```python
from build123d import *

# Parameters (mm, degrees)
SKETCH_1_R      = 1.5
SKETCH_1_R_2    = 1
EXTRUDE_1_DEPTH = 2


with BuildPart() as part:
    # 草图1 → 凸台-拉伸1 (new body)
    with BuildSketch(Plane.XY):
        with BuildLine():
            Line((107.302513423, -106.329977447), (101.737876551, -109.126595767))
            ThreePointArc((101.737876551, -109.126595767), (100.241041238, -109.247857431), (99.081776454, -108.293223729))
            ThreePointArc((99.081776454, -108.293223729), (96.076157143, -102.895430459), (92.952174798, -97.565265927))
            ThreePointArc((92.952174798, -97.565265927), (92.67119221, -96.396525563), (93.110928625, -95.277804356))
            ThreePointArc((93.110928625, -95.277804356), (93.386262354, -90.634283432), (89.082079375, -88.870167754))
            ThreePointArc((89.082079375, -88.870167754), (87.883298953, -88.781676215), (86.951761021, -88.02197737))
            ThreePointArc((86.951761021, -88.02197737), (63.249240179, -56.927091802), (35.446375502, -29.437055089))
            ThreePointArc((35.446375502, -29.437055089), (34.93756912, -29.118601809), (34.357184804, -28.965466337))
            ThreePointArc((34.357184804, -28.965466337), (31.162596189, -27.612410648), (29.250996223, -24.717252331))
            ThreePointArc((29.250996223, -24.717252331), (28.99483955, -24.174407799), (28.589143834, -23.732019493))
            ThreePointArc((28.589143834, -23.732019493), (13.863721442, -12.651321704), (-1.558710581, -2.56328331))
            ThreePointArc((-1.558710581, -2.56328331), (-2.630799159, 1.441837641), (1.322046154, 2.692989782))
            ThreePointArc((1.322046154, 2.692989782), (17.996215952, -6.326789823), (33.906457747, -16.634484455))
            ThreePointArc((33.906457747, -16.634484455), (34.447529327, -16.904338105), (35.04451896, -17.000165164))
            ThreePointArc((35.04451896, -17.000165164), (38.553058948, -18.165150249), (40.712715331, -21.16563811))
            ThreePointArc((40.712715331, -21.16563811), (40.982462328, -21.706762868), (41.401593445, -22.142547854))
            ThreePointArc((41.401593445, -22.142547854), (79.427798672, -58.499548545), (108.618618094, -102.268485529))
            ThreePointArc((108.618618094, -102.268485529), (108.809267395, -104.574248701), (107.302513423, -106.329977447))
        make_face()
        Circle(SKETCH_1_R, mode=Mode.SUBTRACT)
        with Locations((105.955364791, -103.64945687)):
            Circle(SKETCH_1_R_2, mode=Mode.SUBTRACT)
        with Locations((101.955364791, -106.64945687)):
            Circle(SKETCH_1_R_2, mode=Mode.SUBTRACT)
        with Locations((35, -23)):
            Circle(SKETCH_1_R, mode=Mode.SUBTRACT)
    extrude(amount=EXTRUDE_1_DEPTH)


solid = part.part
```
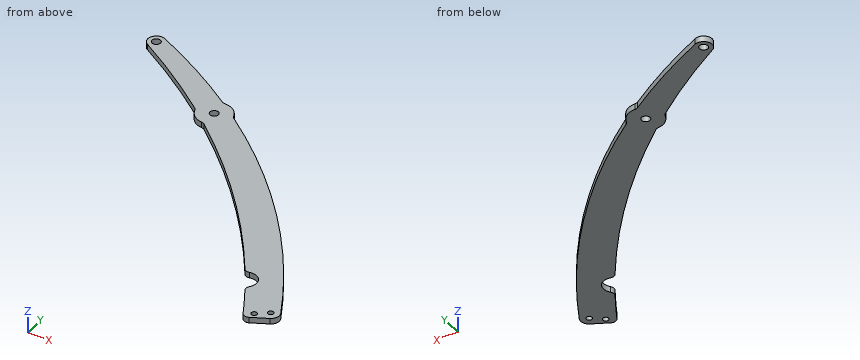
Here's how the part is built. I have some questions about the finished solid (model axes, mm). Round coordinates to 2 decimals unless told otherwise and drop trailing zeros. Loops run counter-clockwise (first coordinate to the right, second up) from the corner with the lowest first, then second, coordinate; pieces in that order, holes last.
1. Suppose I cut it at A-A, the plane z = 1.4. Please give me the cut outline in (x, y) (3 decimals), and give its area (3 significant figures).
Answers:
outline: (-1.559, -2.563) arc R280 cw to (28.589, -23.732) arc R2 cw to (29.251, -24.717) arc R6 ccw to (34.357, -28.965) arc R2 cw to (35.446, -29.437) arc R280 cw to (86.952, -88.022) arc R2 ccw to (89.082, -88.87) arc R4 cw to (93.111, -95.278) arc R2 ccw to (92.952, -97.565) arc R280 cw to (99.082, -108.293) arc R2 ccw to (101.738, -109.127) - (107.303, -106.33) arc R3 ccw to (108.619, -102.268) arc R240 ccw to (41.402, -22.143) arc R2 cw to (40.713, -21.166) arc R6 ccw to (35.045, -17) arc R2 cw to (33.906, -16.634) arc R240 ccw to (1.322, 2.693) arc R3 ccw to start; hole circle Ø3 at (0, 0); hole circle Ø3 at (35, -23); hole circle Ø2 at (101.955, -106.649); hole circle Ø2 at (105.955, -103.649)
area: 1,510 mm2
2. Suppose I cut it at C-C, the plane x = 0. Please give me the cut outline in (y, z).
Answers:
outline: (-3.52, 0) - (-1.5, 0) - (-1.5, 2) - (-3.52, 2) - close; (1.5, 0) - (3, 0) - (3, 2) - (1.5, 2) - close
3. Suppose I cut it at D-D, the plane y = -63. Please give me the cut outline in (x, z).
Answers:
outline: (68.44, 0) - (83.11, 0) - (83.11, 2) - (68.44, 2) - close
4. Will this pin go through, and if not, where does the flat tip stop? pin 1 (1 mm diameter, centred on y = -22.5, z = 1.5, fed in from +X).
Answers:
pin 1: stops at x = 42.52
5. If I drill on probe 1 along Y at (x, z) = (0, 1.3); probe 2 along Y at (x, z) = (35, 1); probe 3 along X at (y, z) = (-22, 1.75), over which ranges is the centre line in solid material (lowest first)?
Answers:
probe 1: y = -3.52 to -1.5, 1.5 to 3
probe 2: y = -29.15 to -24.5, -21.5 to -17
probe 3: x = 26.42 to 33.88, 36.12 to 41.24
6. Suppose I cut it at B-B, the plane y = 0. Please give me the cut outline in (x, z), and give its area (3 significant figures).
Answers:
outline: (-3, 0) - (-1.5, 0) - (-1.5, 2) - (-3, 2) - close; (1.5, 0) - (6.64, 0) - (6.64, 2) - (1.5, 2) - close
area: 13.3 mm2
